Geometry: final body of the model. Coordinates: model frame, mm. A direction names the side the tool comes from. Round coordinates to 2 decimals unless told otherwise and drop trailing zeros. Loops run counter-clockwise (first coordinate to the right, second up) from the corner with the lowest first, then second, coordinate; pieces in that order, holes last. Notation, with made-up numbers: (-11, -26) - (38, -26) arc R10 ccw to (38, -13) - close; hole circle Ø10 at (51, -31). An arc over 180 degrees is marked (long way). Answer as CSV lines item,"result".
from build123d import *

# Parameters (mm, degrees)
EXTRUDE_1_DEPTH     = 2
FILLET_1_R          = 20
SKETCH_3_R          = 2
CUT_EXTRUDE_2_DEPTH = 10
SKETCH_4_R          = 20
CUT_EXTRUDE_3_DEPTH = 10
FILLET_2_R          = 5


with BuildPart() as part:
    # 草图1 → 凸台-拉伸1 (new body)
    with BuildSketch(Plane.XY):
        Polygon((110, 45.563491861), (45.563491861, 110), (-45.563491861, 110), (-110, 45.563491861), (-110, -45.563491861), (-45.563491861, -110), (45.563491861, -110), (110, -45.563491861), align=None)
    extrude(amount=EXTRUDE_1_DEPTH)

    # 圆角1
    fillet_1_edges = [part.edges().sort_by_distance(p)[0] for p in [
        (110, -45.563491861, 1),
        (45.563491861, -110, 1),
        (-45.563491861, -110, 1),
        (-110, -45.563491861, 1),
        (-110, 45.563491861, 1),
        (-45.563491861, 110, 1),
        (45.563491861, 110, 1),
        (110, 45.563491861, 1),
    ]]
    fillet(fillet_1_edges, radius=FILLET_1_R)

    # 草图3 → 切除-拉伸2 (cut)
    with BuildSketch(Plane(origin=(0, 0, 0), x_dir=(-1, 0, 0), z_dir=(0, 0, -1))):
        with Locations((-99.317049745, 41.138468979)):
            Circle(SKETCH_3_R)
        with Locations((-41.138468979, 99.317049745)):
            Circle(SKETCH_3_R)
        with Locations((41.138468979, 99.317049745)):
            Circle(SKETCH_3_R)
        with Locations((99.317049745, 41.138468979)):
            Circle(SKETCH_3_R)
        with Locations((99.317049745, -41.138468979)):
            Circle(SKETCH_3_R)
        with Locations((41.138468979, -99.317049745)):
            Circle(SKETCH_3_R)
        with Locations((-41.138468979, -99.317049745)):
            Circle(SKETCH_3_R)
        with Locations((-99.317049745, -41.138468979)):
            Circle(SKETCH_3_R)
    extrude(amount=-CUT_EXTRUDE_2_DEPTH, mode=Mode.SUBTRACT)

    # 草图4 → 切除-拉伸3 (cut)
    with BuildSketch(Plane(origin=(0, 0, 0), x_dir=(-1, 0, 0), z_dir=(0, 0, -1))):
        Circle(SKETCH_4_R)
        Polygon((88.053996306, 25.913196146), (44.857355713, 80.08007017), (19.545787062, 15.587245046), align=None)
        Polygon((0, 25), (34.641016151, 85), (-34.641016151, 85), align=None)
        Polygon((75.160521268, -52.686772939), (90.577223803, 14.858214166), (24.373197805, -5.563023349), align=None)
        Polygon((5.66964072, -91.612527386), (68.09059493, -61.552180157), (10.847093478, -22.524221698), align=None)
        Polygon((-68.09059493, -61.552180157), (-5.66964072, -91.612527386), (-10.847093478, -22.524221698), align=None)
        Polygon((-90.577223803, 14.858214166), (-75.160521268, -52.686772939), (-24.373197805, -5.563023349), align=None)
        Polygon((-44.857355713, 80.08007017), (-88.053996306, 25.913196146), (-19.545787062, 15.587245046), align=None)
    extrude(amount=-CUT_EXTRUDE_3_DEPTH, mode=Mode.SUBTRACT)

    # 圆角2
    fillet_2_edges = [part.edges().sort_by_distance(p)[0] for p in [
        (0, 25, 1),
        (34.641016151, 85, 1),
        (-34.641016151, 85, 1),
        (-5.66964072, -91.612527386, 1),
        (-10.847093478, -22.524221698, 1),
        (-68.09059493, -61.552180157, 1),
        (68.09059493, -61.552180157, 1),
        (10.847093478, -22.524221698, 1),
        (5.66964072, -91.612527386, 1),
        (90.577223803, 14.858214166, 1),
        (24.373197805, -5.563023349, 1),
        (75.160521268, -52.686772939, 1),
        (44.857355713, 80.08007017, 1),
        (19.545787062, 15.587245046, 1),
        (88.053996306, 25.913196146, 1),
        (-88.053996306, 25.913196146, 1),
        (-19.545787062, 15.587245046, 1),
        (-44.857355713, 80.08007017, 1),
        (-75.160521268, -52.686772939, 1),
        (-24.373197805, -5.563023349, 1),
        (-90.577223803, 14.858214166, 1),
    ]]
    fillet(fillet_2_edges, radius=FILLET_2_R)


solid = part.part
(1) Pin query (flat end, axial travel): P1, Ø4.5, axis at x = -99.32, y = -41.14, coming from the +Z side; P2, Ø1, axis at y = 78.5, z = 1, coming from the -X side. Return the tip coordinate at first contact, or that it passes through.
Findings below:
P1,"z = 2"
P2,"x = -77.56"
(2) Section B-B (y = 0). Output: boundary loops of the cut face in (x, z), and give its area (3 significant figures).
Findings below:
outline,"(-110, 0) - (-87.19, 0) - (-87.19, 2) - (-110, 2) - close; (-42.41, 0) - (-20, 0) - (-20, 2) - (-42.41, 2) - close; (20, 0) - (42.41, 0) - (42.41, 2) - (20, 2) - close; (87.19, 0) - (110, 0) - (110, 2) - (87.19, 2) - close"
area,"181 mm2"
(3) Section A-A (x = 0). Output: boundary loops of the cut face in (y, z), and give its area (3 significant figures).
Findings below:
outline,"(-110, 0) - (-20, 0) - (-20, 2) - (-110, 2) - close; (20, 0) - (30, 0) - (30, 2) - (20, 2) - close; (85, 0) - (110, 0) - (110, 2) - (85, 2) - close"
area,"250 mm2"
(4) Section D-D (z = 0.85). Give the number of separate pieces and of enclosed holes in the cut face, and give its area (3 significant figures).
Findings below:
separate pieces,"1"
enclosed holes,"16"
area,"24,500 mm2"
(5) Access query for faces 5 (the face through (-32.334, 48.172, 0.986)), 6 (the face through (-2, -23, 2)). Directions: +Z, -Z, +X, -X, +Y, -Y. A direction counts if a zero-diameter tool reaches every point of the face in a straight line with its end or side. Return the directions, or none.
Findings below:
face 5,"+Z, -Z"
face 6,"+Z, +X, -X, +Y, -Y"
(6) Material intervals for line 1 along X through (y, z) = (-82, 1.4); line 2 along Y through (x, z) = (-60, 1.5); line 3 along X through (y, z) = (-23, 1.6), sorted ascending.
Findings below:
line 1,"-73.56 to -25.63, -6.39 to 6.39, 25.63 to 73.56"
line 2,"-95.56 to -65.45, -56.04 to -38.62, 5.43 to 21.68, 61.09 to 95.56"
line 3,"-110 to -81.94, -43.17 to 43.17, 81.94 to 110"
(7) Draft query along Y for faces 1 (the face through (77.413, -78.151, 0.986)), 2 (the face through (45.034, 108.435, 1.014)), 3 (the face through (-2, -23, 0)), 4 (the face through (-17.14, 54.69, 0.99)). Return one class per face: pulls with the +Y half, pulls with the -Y half, needs draft (parallel to the pull), parting line crosses it, or undercut.
Findings below:
face 1,"pulls with the -Y half"
face 2,"pulls with the +Y half"
face 3,"needs draft"
face 4,"undercut"
(8) Section C-C (x = 47.5). Output: boundary loops of the cut face in (y, z).
Findings below:
outline,"(-107.19, 0) - (-71.47, 0) - (-71.47, 2) - (-107.19, 2) - close; (-47.51, 0) - (-27.02, 0) - (-27.02, 2) - (-47.51, 2) - close; (1.57, 0) - (19.8, 0) - (19.8, 2) - (1.57, 2) - close; (75.06, 0) - (107.19, 0) - (107.19, 2) - (75.06, 2) - close"
